Design review of the part built by this model. Coordinates are the model's own, in mm. A direction names the side the tool comes from. Give positions to 0.01 mm unless a question says otherwise; leave off trailing zeros. Write each loop counter-clockwise with the first axis right and the second up, starting at its lowest first coordinate (ties: lowest second). Pieces come first, ordered by that corner, then holes. Notation, with made-up numbers: M 17,53 L 74,53 A11 cw 74,57 Z; hole C 72.25,45.5 d3. An arc over 180 degrees is marked long. Use a Markdown table: item, result. Add a question column.
```python
from build123d import *

# Parameters (mm, degrees)
F0_W     = 117
F0_H     = 77
F0_R     = 3.5
F0_R_2   = 1.25
F1_DEPTH = 3
F2_DEPTH = 10


with BuildPart() as f1:
    # F0 (on Top) → F1 (new body)
    with BuildSketch(Plane.XY):
        with Locations((1.2832747996, -1.2006596088)):
            Rectangle(F0_W, F0_H)
        with Locations((-40.9167252004, -24.7006596088)):
            Circle(F0_R, mode=Mode.SUBTRACT)
        with Locations((24.7832747996, -29.7006596088)):
            Circle(F0_R, mode=Mode.SUBTRACT)
        with Locations((54.7832747996, -29.7006596088)):
            Circle(F0_R, mode=Mode.SUBTRACT)
        with Locations((11.0832747996, -19.6006596088)):
            Circle(F0_R, mode=Mode.SUBTRACT)
        with Locations((-39.7167252004, 23.4993403912)):
            Circle(F0_R, mode=Mode.SUBTRACT)
        with Locations((11.0832747996, 8.2993403912)):
            Circle(F0_R, mode=Mode.SUBTRACT)
        with Locations((24.7832747996, 27.2993403912)):
            Circle(F0_R, mode=Mode.SUBTRACT)
        with Locations((54.7832747996, 27.2993403912)):
            Circle(F0_R, mode=Mode.SUBTRACT)
        with Locations((-39.7167252004, 23.4993403912)):
            Circle(F0_R)
        with Locations((-39.7167252004, 23.4993403912)):
            Circle(F0_R_2, mode=Mode.SUBTRACT)
        with Locations((11.0832747996, 8.2993403912)):
            Circle(F0_R)
        with Locations((11.0832747996, 8.2993403912)):
            Circle(F0_R_2, mode=Mode.SUBTRACT)
        with Locations((11.0832747996, -19.6006596088)):
            Circle(F0_R)
        with Locations((11.0832747996, -19.6006596088)):
            Circle(F0_R_2, mode=Mode.SUBTRACT)
        with Locations((-40.9167252004, -24.7006596088)):
            Circle(F0_R)
        with Locations((-40.9167252004, -24.7006596088)):
            Circle(F0_R_2, mode=Mode.SUBTRACT)
        with Locations((24.7832747996, 27.2993403912)):
            Circle(F0_R)
        with Locations((24.7832747996, 27.2993403912)):
            Circle(F0_R_2, mode=Mode.SUBTRACT)
        with Locations((54.7832747996, 27.2993403912)):
            Circle(F0_R)
        with Locations((54.7832747996, 27.2993403912)):
            Circle(F0_R_2, mode=Mode.SUBTRACT)
        with Locations((54.7832747996, -29.7006596088)):
            Circle(F0_R)
        with Locations((54.7832747996, -29.7006596088)):
            Circle(F0_R_2, mode=Mode.SUBTRACT)
        with Locations((24.7832747996, -29.7006596088)):
            Circle(F0_R)
        with Locations((24.7832747996, -29.7006596088)):
            Circle(F0_R_2, mode=Mode.SUBTRACT)
        with Locations((11.0832747996, 8.2993403912)):
            Circle(F0_R_2)
        with Locations((11.0832747996, -19.6006596088)):
            Circle(F0_R_2)
        with Locations((-40.9167252004, -24.7006596088)):
            Circle(F0_R_2)
        with Locations((-39.7167252004, 23.4993403912)):
            Circle(F0_R_2)
        with Locations((24.7832747996, 27.2993403912)):
            Circle(F0_R_2)
        with Locations((54.7832747996, 27.2993403912)):
            Circle(F0_R_2)
        with Locations((54.7832747996, -29.7006596088)):
            Circle(F0_R_2)
        with Locations((24.7832747996, -29.7006596088)):
            Circle(F0_R_2)
    extrude(amount=-F1_DEPTH)

    # F0 (on Top) → F2 (join)
    with BuildSketch(Plane.XY):
        with Locations((-39.7167252004, 23.4993403912)):
            Circle(F0_R)
        with Locations((-39.7167252004, 23.4993403912)):
            Circle(F0_R_2, mode=Mode.SUBTRACT)
        with Locations((11.0832747996, 8.2993403912)):
            Circle(F0_R)
        with Locations((11.0832747996, 8.2993403912)):
            Circle(F0_R_2, mode=Mode.SUBTRACT)
        with Locations((11.0832747996, -19.6006596088)):
            Circle(F0_R)
        with Locations((11.0832747996, -19.6006596088)):
            Circle(F0_R_2, mode=Mode.SUBTRACT)
        with Locations((-40.9167252004, -24.7006596088)):
            Circle(F0_R)
        with Locations((-40.9167252004, -24.7006596088)):
            Circle(F0_R_2, mode=Mode.SUBTRACT)
        with Locations((24.7832747996, -29.7006596088)):
            Circle(F0_R)
        with Locations((24.7832747996, -29.7006596088)):
            Circle(F0_R_2, mode=Mode.SUBTRACT)
        with Locations((54.7832747996, -29.7006596088)):
            Circle(F0_R)
        with Locations((54.7832747996, -29.7006596088)):
            Circle(F0_R_2, mode=Mode.SUBTRACT)
        with Locations((24.7832747996, 27.2993403912)):
            Circle(F0_R)
        with Locations((24.7832747996, 27.2993403912)):
            Circle(F0_R_2, mode=Mode.SUBTRACT)
        with Locations((54.7832747996, 27.2993403912)):
            Circle(F0_R)
        with Locations((54.7832747996, 27.2993403912)):
            Circle(F0_R_2, mode=Mode.SUBTRACT)
    extrude(amount=F2_DEPTH)


solid = f1.part
```
(1) Add section C-C on y = -3. Give the boundary of the cut face in (x, z).
(2) The part is to be moulded in two halves that separate along Y. For faces 1 (the flat face through (11, 6.8, 10)), 2 (the cylindrical face through (-36.38, 24.55, 4.93)), say which applies: released by +Y, released by -Y, zero draft, split by the parting line, or undercut.
(3) Add section B-B on x = -26.5. Give the boundary of the cut face in (y, z).
(4) Add section A-A on z = 6. Give the number of separate pieces and of enclosed holes in the cut face, then the cut area to 3 significant figures.
(5) Machinability: for faces 3 (the cylindrical face through (24.62, -28.46, 4.93)), 4 (the flat face through (0, -1, -3)), which of the approach directions +Z, -Z, +X, -X, +Y, -Y give a long, thin tool a straight path to every point of the face, cutting with its end or side? Answer none if there is none.
(6) Wall thickness on L1, parallel to Y at x = -41, z = 8.75; L2, parallel to Z at x = -18, y = 18; L3, parallel to X at y = 30.5, z = 6.25: over which ranges is each line inside the solid? List them lowest first.
(7) For pin 1 (1.2 mm diameter, centred on x = -39.5, y = 23, fed in from +Z); pin 2 (1.5 mm diameter, centred on x = -37.5, z = 7, fed in from -Y); pin 3 (3 mm diameter, centred on x = 24, y = 27, fed in from +Z); pin 4 (4 mm diameter, centred on x = 10.5, z = 7, fed in from +Y), all flat-tipped, find the tip position at first contact; note any pin that passes through.
From the geometry:
| question | item | result |
|---|---|---|
| 1 | outline | M -57.22,-3 L 59.78,-3 L 59.78,0 L -57.22,0 Z |
| 2 | face 1 | zero draft |
| 2 | face 2 | undercut |
| 3 | outline | M -39.7,-3 L 37.3,-3 L 37.3,0 L -39.7,0 Z |
| 4 | separate pieces | 8 |
| 4 | enclosed holes | 8 |
| 4 | area | 269 mm^2 |
| 5 | face 3 | +Z |
| 5 | face 4 | -Z, +X, -X, +Y, -Y |
| 6 | L1 | y = -28.2 to -25.95, -23.45 to -21.2, 20.24 to 26.76 |
| 6 | L2 | z = -3 to 0 |
| 6 | L3 | x = 23.37 to 26.2, 53.37 to 56.2 |
| 7 | pin 1 | stops at z = 0 |
| 7 | pin 2 | stops at y = -26.97 |
| 7 | pin 3 | stops at z = 10 |
| 7 | pin 4 | stops at y = 11.8 |
